Verification items for the finished model (mm, model axes). A direction names the side the tool comes from. Round coordinates to 2 decimals unless told otherwise and drop trailing zeros. Write each loop counter-clockwise with the first axis right and the second up, starting at its lowest first coordinate (ties: lowest second). Pieces come first, ordered by that corner, then holes. Notation, with made-up numbers: M -6,41 L 53,41 A18 cw 53,67 Z; hole C -39,89 d4. An arc over 180 degrees is marked long. One line per question, with ' | ' between items. Start each with the question number.
Q1. Cross-section at A-A (y = -15). Record the boundary of the cut face in (x, z), then the cut area to 3 significant figures.
Q2. Thickness scan on line 1 along X through (y, z) = (-4, 0); line 2 along X through (y, z) = (-3.5, -12.5); line 3 along Z through (x, y) = (26, 13). Record the ranges inside material, lowest first. Write a range as from..to.
Q3. Tool access check on faces 4 (the face through (-0.65, -17.93, 37.47)), 5 (the face through (39.05, -7.32, 8.67)), 6 (the face through (21, -10, 28)). Record the directions out of +Z, -Z, +X, -X, +Y, -Y that give a thin tool (end or side, any length) a straight path to the whole face; none if there is none.
Q4. Release check for a two-part mould opening along Y. For faces 1 (the face through (0, 30, 0)), 2 (the face through (-33.144, -17.662, -17.537)), 3 (the face through (0, 22.929, 0)) record: released by +Y, released by -Y, zero draft, split by the parting line, or undercut.
Q5. Gauge pin test, flat ends, axial feed: pin 1 (1 mm diameter, centred on x = -16, y = 17.5, fed in from -Z); pin 2 (2 mm diameter, centred on x = 3.5, z = 29, fed in from +Y); pin 3 (12 mm diameter, centred on x = -0.5, z = -3.5, fed in from -Y). Record the tip position at first contact, or that the pin passes through.
from build123d import *

# Parameters (mm, degrees)
CUT_EXTRUDE1_REACH      = 96.34
CUT_EXTRUDE1_END_RADIUS = 35
SKETCH2_R               = 3
CIRPATTERN1_COUNT       = 3


with BuildPart() as part:
    # Sketch1 → Revolve1 (revolve)
    with BuildSketch(Plane.XY, mode=Mode.PRIVATE) as revolve1_sk:
        with BuildLine():
            Line((-20, 30), (0, 30))
            Line((0, 30), (0, 22.928932188))
            Line((0, 22.928932188), (-20, 22.928932188))
            add(Edge.make_bspline(
                [(-20, 22.928932188), (-32.99251078, 14.579736434), (-35, 0)],
                knots=[0, 0, 0, 1, 1, 1], degree=2))
            Line((-35, 0), (-35, -20))
            Line((-35, -20), (-40, -20))
            Line((-40, -20), (-40, 0))
            Line((-40, 0), (-40, 5))
            add(Edge.make_bspline(
                [(-20, 30), (-35.448934618, 21.981430701), (-40, 5)],
                knots=[0, 0, 0, 1, 1, 1], degree=2))
        make_face()
    revolve(revolve1_sk.sketch.rotate(Axis((0, -63.953488372, 0), (0, 1, 0)), 270), axis=Axis((0, -63.953488372, 0), (0, 1, 0)))

    # Cut-Extrude1: up to this cylinder (the profile starts outside it)
    cut_extrude1_end = Plane(origin=(0, -15, 0), z_dir=(0, -1, 0)) * Cylinder(CUT_EXTRUDE1_END_RADIUS, 263.68, mode=Mode.PRIVATE)
    # Sketch2 → Cut-Extrude1 (cut, up to the surface)
    with BuildSketch(Plane.XY.offset(40), mode=Mode.PRIVATE) as cut_extrude1_sk1:
        with Locations((0, -15)):
            Circle(SKETCH2_R)
    cut_extrude1_tool1 = extrude(cut_extrude1_sk1.sketch, amount=-CUT_EXTRUDE1_REACH, mode=Mode.PRIVATE) - cut_extrude1_end
    cut_extrude1 = cut_extrude1_tool1.solids().sort_by_distance((0, -15, 40))[0]
    add(cut_extrude1, mode=Mode.SUBTRACT)

    # CirPattern1: Cut-Extrude1 ×3 about axis
    cirpattern1_axis = Axis((0, 5, 0), (0, -1, 0))
    for i in range(1, CIRPATTERN1_COUNT):
        add(cut_extrude1.rotate(cirpattern1_axis, i * 360 / CIRPATTERN1_COUNT), mode=Mode.SUBTRACT)


solid = part.part
Determined:
1) outline: M -36.04,-17.35 L -31.7,-14.84 A35 cw -3,34.87 L -3,39.89 A40 ccw Z; M -33.04,-22.54 A40 ccw 33.04,-22.54 L 28.7,-20.03 A35 cw -28.7,-20.03 Z; M 3,34.87 A35 cw 31.7,-14.84 L 36.04,-17.35 A40 ccw 3,39.89 Z | area: 1,090 mm²
2) line 1: x = -40..-35, 35..40 | line 2: x = -38..-32.69, 32.69..38 | line 3: z = -26.34..-15.48, 15.48..26.34
3) face 4: +Z | face 5: +Y, -Y | face 6: -Y
4) face 1: released by +Y | face 2: undercut | face 3: released by -Y
5) pin 1: stops at z = -30.89 | pin 2: stops at y = 24.45 | pin 3: stops at y = 22.93
